Source: three-view drawing plus pictorial views. Frame: mm from the lowest corner of the part. A direction names the side the tool comes from. Round coordinates to 2 decimals unless told otherwise and drop trailing zeros. Loops run counter-clockwise (first coordinate to the right, second up) from the corner with the lowest first, then second, coordinate; pieces in that order, holes last. Notation, with made-up numbers: M -31,74.25 L 23,74.25 A18 cw 23,101.25 Z; hole C 4,0 d5. An arc over 180 degrees is marked long. Answer as a JSON object with one key per item and string values.
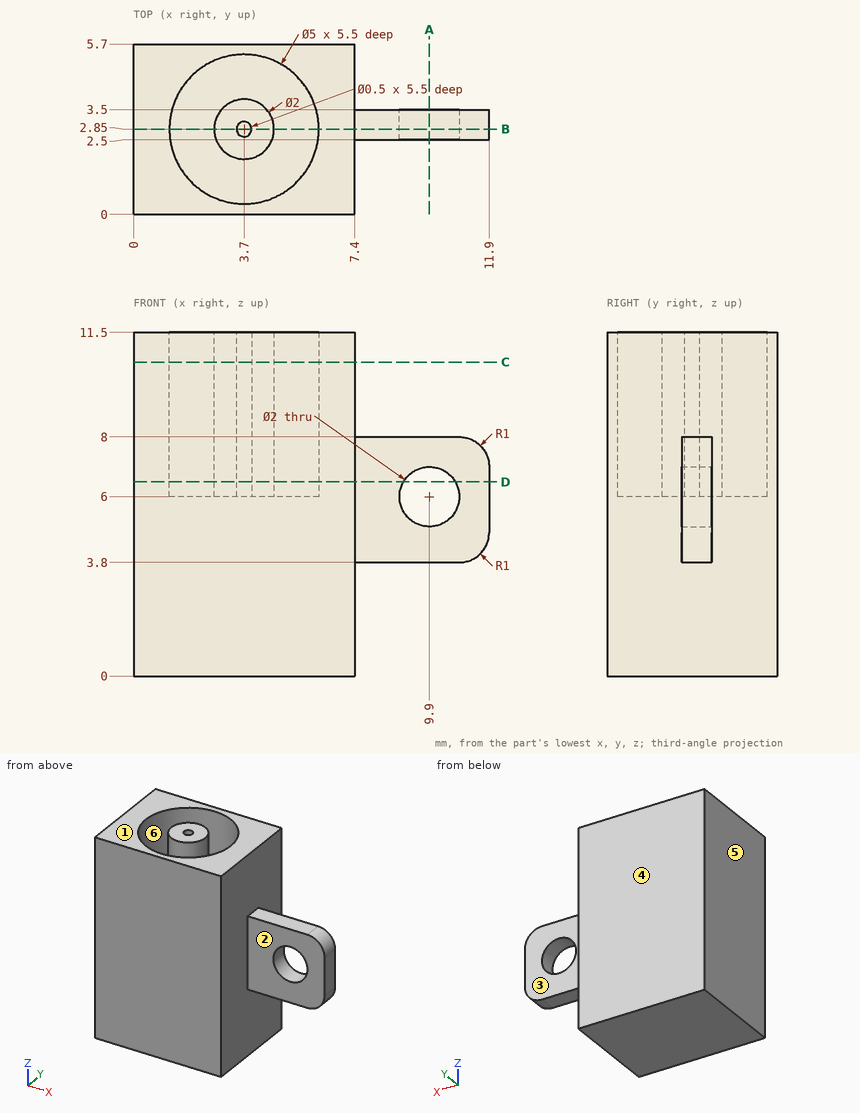
1) Cut plane B-B on y = 2.85. Return the cut outline in (x, z).
Geometry results:
{"outline": "M 0,0 L 7.4,0 L 7.4,3.8 L 10.9,3.8 A1 ccw 11.9,4.8 L 11.9,7 A1 ccw 10.9,8 L 7.4,8 L 7.4,11.5 L 6.2,11.5 L 6.2,6 L 4.7,6 L 4.7,11.5 L 3.95,11.5 L 3.95,6 L 3.45,6 L 3.45,11.5 L 2.7,11.5 L 2.7,6 L 1.2,6 L 1.2,11.5 L 0,11.5 Z; hole C 9.9,6 d2"}
2) Cut plane D-D on z = 6.5. Return the cut outline in (x, y), and give its area (3 significant figures).
Geometry results:
{"outline": "M 0,0 L 7.4,0 L 7.4,2.5 L 9.03,2.5 L 9.03,3.5 L 7.4,3.5 L 7.4,5.7 L 0,5.7 Z; C 3.7,2.85 d2; M 10.77,2.5 L 11.9,2.5 L 11.9,3.5 L 10.77,3.5 Z; hole C 3.7,2.85 d5; hole C 3.7,2.85 d0.5", "area": "28.3 mm2"}
3) Set-up query: the marked faces 1, 2 and 3. Return all of +Z, -Z, +X, -X, +Y, -Y with unobstructed straight access to the full face (end or side cutting, diameter ignored); none if empty.
Geometry results:
{"face 1": "+Z, +X, -X, +Y, -Y", "face 2": "+Z, -Z, +X, -Y", "face 3": "+Z, -Z, +X, +Y"}
4) Pull-direction query (X, two-part tool) for the marked faces 4, 5 and 6; classes: +X half, -X half, draft (parallel to the pull), parting line (faces both ways), or undercut.
Geometry results:
{"face 4": "draft", "face 5": "-X half", "face 6": "undercut"}
5) Cut plane C-C on z = 10.5. Return the cut outline in (x, y), and give its area (3 significant figures).
Geometry results:
{"outline": "M 0,0 L 7.4,0 L 7.4,5.7 L 0,5.7 Z; C 3.7,2.85 d2; hole C 3.7,2.85 d5; hole C 3.7,2.85 d0.5", "area": "25.5 mm2"}
6) Cut plane A-A on x = 9.9. Return the cut outline in (y, z), and give its area (3 significant figures).
Geometry results:
{"outline": "M 2.5,3.8 L 3.5,3.8 L 3.5,5 L 2.5,5 Z; M 2.5,7 L 3.5,7 L 3.5,8 L 2.5,8 Z", "area": "2.20 mm2"}
7) Line query: probe 1 along Y at (x, z) = (3.7, 10.1); probe 2 along Z at (x, y) = (9.9, 3); probe 3 along X at (y, z) = (3.4, 1.5). Output: solid intervals per line, ascending.
Geometry results:
{"probe 1": "0 to 0.35, 1.85 to 2.6, 3.1 to 3.85, 5.35 to 5.7", "probe 2": "3.8 to 5, 7 to 8", "probe 3": "0 to 7.4"}
8) First-contact query: pin 1 (1.5 mm diameter, centred on x = 9, y = 4.5, fed in from -Z); pin 2 (3 mm diameter, centred on x = 7.5, y = 3, fed in from +Z); pin 3 (1.1 mm diameter, centred on x = 9, y = 3, fed in from -Z); pin 4 (4.5 mm diameter, centred on x = 10.5, z = 5, fed in from +Y). Flat tips, straight axial feed; report the tip coordinate or a pass-through.
Geometry results:
{"pin 1": "through", "pin 2": "z = 11.5", "pin 3": "z = 3.8", "pin 4": "y = 3.5"}
